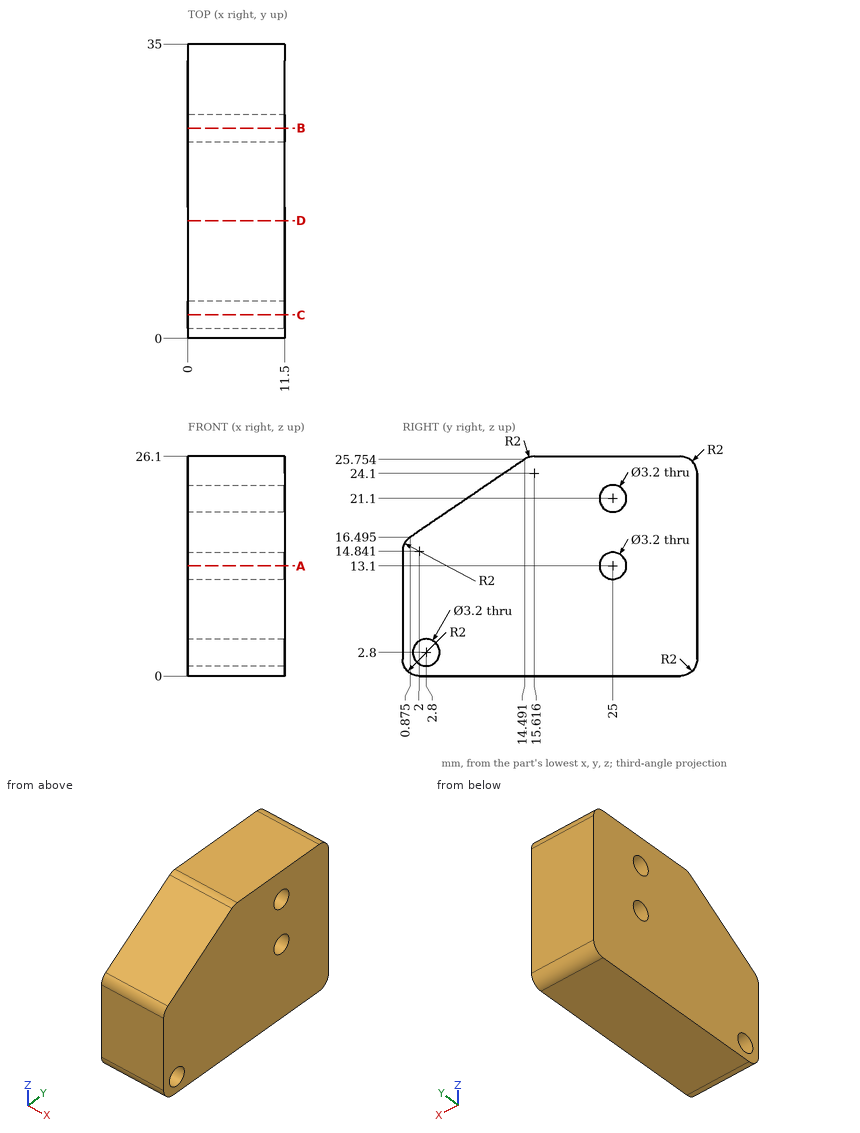
Study the drawing (mm; zero at the part's minimum x, y, z) and answer. Give positions to 0.01 mm unless a question says otherwise; leave off trailing zeros. Order: outer loops, then holes, each group sorted by start corner. A loop starts at its lowest first (then second) coordinate and runs counter-clockwise, first axis right, second up. Notation, with made-up numbers: (-33.75, 79.5) - (-3.75, 79.5) arc R19 cw to (-3.75, 91.5) - close; hole circle Ø10 at (-15.75, -23.75). An arc over 180 degrees is marked (long way). Answer as CSV lines item,"result". Start each with the question number.
Q1. The part is cut by section D-D (y = 14). Write down the section's boundary in (x, z).
Q2. The part is cut by section B-B (y = 25). Write down the section's boundary in (x, z).
Q3. Given pin 1 Ø3 at (x, z) = (5.5, 13.5) entering from -Y; pin 2 Ø1.5 at (x, y) = (7, 8.5) entering from +Z; pin 3 Ø4 at (x, y) = (9.5, 4.5) entering from +Z, each flat-ended and moving along its own axis, determine where each tip first touches the part or whether it passes through.
Q4. The part is cut by section C-C (y = 2.8). Write down the section's boundary in (x, z), then the cut area to 3 significant figures.
Q5. The part is cut by section A-A (z = 13.1). Write down the section's boundary in (x, y), then the cut area to 3 significant figures.
Q6. Find the intervals of material crossed by L1, parallel to Z at x = 6, y = 25; L2, parallel to Z at x = 8, y = 25.5; L3, parallel to Z at x = 8.5, y = 3.5, in increasing order. Write a range as [from, to].
Check result:
1,outline,"(0, 0) - (11.5, 0) - (11.5, 25.42) - (0, 25.42) - close"
2,outline,"(0, 0) - (11.5, 0) - (11.5, 11.5) - (0, 11.5) - close; (0, 14.7) - (11.5, 14.7) - (11.5, 19.5) - (0, 19.5) - close; (0, 22.7) - (11.5, 22.7) - (11.5, 26.1) - (0, 26.1) - close"
3,pin 1,"stops at y = 0"
3,pin 2,"stops at z = 22.19"
3,pin 3,"stops at z = 20.32"
4,outline,"(0, 0) - (11.5, 0) - (11.5, 1.2) - (0, 1.2) - close; (0, 4.4) - (11.5, 4.4) - (11.5, 17.8) - (0, 17.8) - close"
4,area,"168 mm²"
5,outline,"(0, 0) - (11.5, 0) - (11.5, 23.4) - (0, 23.4) - close; (0, 26.6) - (11.5, 26.6) - (11.5, 35) - (0, 35) - close"
5,area,"366 mm²"
6,L1,"z = [0, 11.5], [14.7, 19.5], [22.7, 26.1]"
6,L2,"z = [0, 11.58], [14.62, 19.58], [22.62, 26.1]"
6,L3,"z = [0, 1.36], [4.24, 18.28]"
